Geometry check sheet. Reference: drawing and pictorial views, mm from the part's lowest x, y, z. Round coordinates to 2 decimals unless told otherwise and drop trailing zeros. Loops run counter-clockwise (first coordinate to the right, second up) from the corner with the lowest first, then second, coordinate; pieces in that order, holes last. Notation, with made-up numbers: M -23,42 L -13,42 A23 cw -13,66 Z; hole C -36,-10.5 d10. An arc over 180 degrees is marked long. One line per question, with ' | ' between items. Start each with the question number.
(1) Go/stop test with a flat-tipped pin: P1, Ø6, axis at x = 8, y = 11.5, coming from the +Z side. Record where the tip stops, or that it passes through.
(2) Section check C-C (y = 9.75). Record the boundary of the cut face in (x, z).
(3) Section check A-A (x = 14.5). Record the boundary of the cut face in (y, z) (1 decimal), and give its area (3 significant figures).
(4) Thickness scan on probe 1 along Z at (x, y) = (10.5, 7.75); probe 2 along Z at (x, y) = (7, 6.25); probe 3 along Y at (x, z) = (9, 22.5) (1 decimal). Record the ranges inside material, lowest first. Write a range as [from, to].
(5) Section check B-B (z = 20.75). Record the boundary of the cut face in (x, y).
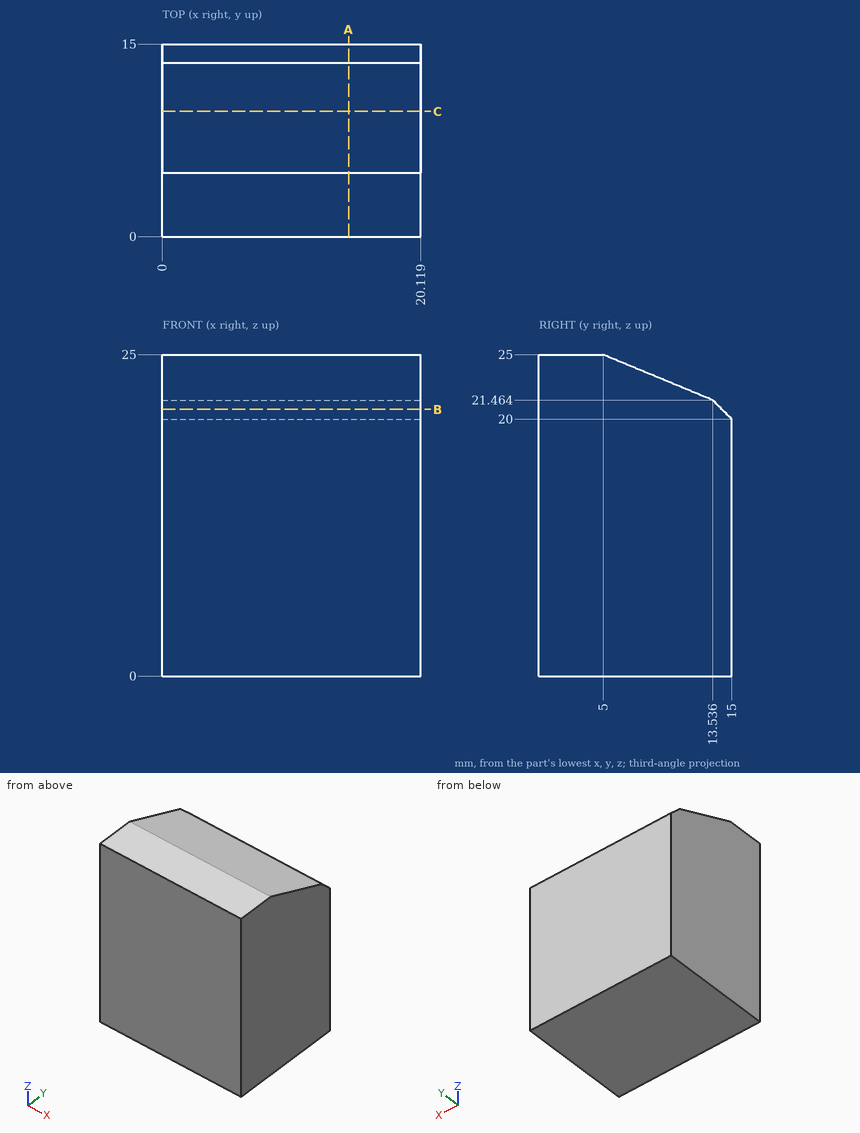
The answers:
1) P1: z = 23.55
2) outline: M 0,0 L 20.12,0 L 20.12,23.03 L 0,23.03 Z
3) outline: M 0,0 L 15,0 L 15,20 L 13.5,21.5 L 5,25 L 0,25 Z | area: 354 mm²
4) probe 1: [0, 23.86] | probe 2: [0, 24.48] | probe 3: [0, 11]
5) outline: M 0,0 L 20.12,0 L 20.12,14.25 L 0,14.25 Z
